from build123d import *

# Parameters (mm, degrees)
F0_W      = 84
F0_H      = 84
F1_DEPTH  = 27
F2_T      = -2.5
F3_DEPTH  = 2
F4_W      = 65
F4_H      = 14
F5_DEPTH  = 25
F6_W      = 10
F6_H      = 10
F7_DEPTH  = 21.8
F4_R      = 2
F8_DEPTH  = 25
F9_DEPTH  = 2
F10_R     = 3.5
F10_R_2   = 1.8
F11_DEPTH = 21
F12_DEPTH = 10
F13_R     = 1
F14_DEPTH = 2
F15_R     = 3


# Not quite as in the source:
# - a feature names something its author has since deleted; it is built from what else it names


with BuildPart() as f1:
    # F0 (on Top) → F1 (new body)
    with BuildSketch(Plane.XY):
        Rectangle(F0_W, F0_H)
    extrude(amount=F1_DEPTH)

    # F2
    f2_openings = [f1.faces().sort_by_distance(p)[0] for p in [
        (0, 0, 27),
    ]]
    offset(amount=F2_T, openings=f2_openings)

    # F3 (cut): a face of the model
    f3_faces = [f1.faces().sort_by_distance(p)[0] for p in [
        (0, 0, 2.5),
    ]]
    extrude(f3_faces, amount=F3_DEPTH, mode=Mode.SUBTRACT)

    # F4 (on face) → F5 (cut)
    with BuildSketch(Plane.XY.offset(2.5)):
        with Locations((0, -27)):
            Rectangle(F4_W, F4_H)
    extrude(amount=-F5_DEPTH, mode=Mode.SUBTRACT)

    # F6 (on face) → F7 (cut)
    with BuildSketch(Plane.YZ.offset(42)):
        with Locations((-27, 5)):
            Rectangle(F6_W, F6_H)
    extrude(amount=-F7_DEPTH, mode=Mode.SUBTRACT)

    # F4 (on face) → F8 (cut)
    with BuildSketch(Plane.XY.offset(2.5)):
        with Locations((0, 26.6423244029)):
            Circle(F4_R)
        with Locations((0, -10.8067262918)):
            Circle(F4_R)
    extrude(amount=-F8_DEPTH, mode=Mode.SUBTRACT)

    # F9 (cut): faces of the model
    f9_faces = [f1.faces().sort_by_distance(p)[0] for p in [
        (0, 40.8120606076, 27),
        (-0.4812956241, 5.0155977429, 2.5),
    ]]
    extrude(f9_faces, amount=-F9_DEPTH, mode=Mode.SUBTRACT)

    # F10 (on Top) → F11 (join)
    with BuildSketch(Plane.XY):
        with Locations((-31.5, 0)):
            Circle(F10_R)
        with Locations((-31.5, 0)):
            Circle(F10_R_2, mode=Mode.SUBTRACT)
        with Locations((31.5, 0)):
            Circle(F10_R)
        with Locations((31.5, 0)):
            Circle(F10_R_2, mode=Mode.SUBTRACT)
    extrude(amount=F11_DEPTH)

    # F10 (on Top) → F12 (join)
    with BuildSketch(Plane.XY):
        with Locations((-31.5, 0)):
            Circle(F10_R_2)
        with Locations((31.5, 0)):
            Circle(F10_R_2)
    extrude(amount=F12_DEPTH)

    # F13
    f13_edges = [f1.edges().sort_by_distance(p)[0] for p in [
        (-42, 42, 12.5),
        (42, 42, 12.5),
        (42, -42, 12.5),
        (-42, -42, 12.5),
    ]]
    fillet(f13_edges, radius=F13_R)

    # F14 (add): a face of the model
    f14_faces = [f1.faces().sort_by_distance(p)[0] for p in [
        (-0.5873435355, 4.470699491, 0),
    ]]
    extrude(f14_faces, amount=F14_DEPTH)

    # F15
    f15_edges = [f1.edges().sort_by_distance(p)[0] for p in [
        (-35, 0, 0.5),
        (28, 0, 0.5),
    ]]
    fillet(f15_edges, radius=F15_R)


solid = f1.part
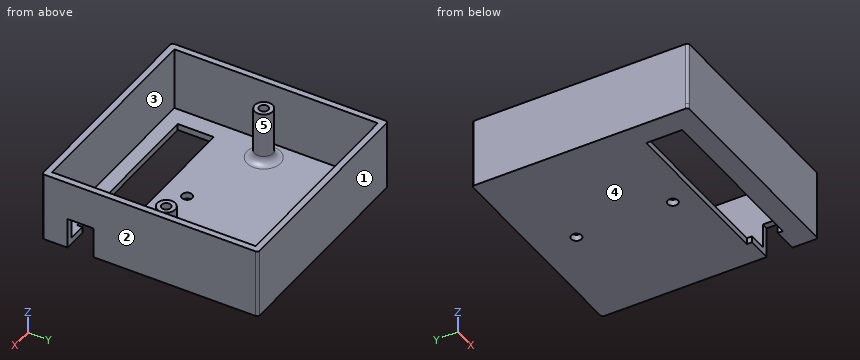
Can you work these out from the model? Positions are in its coordinate system, mm. Face numbers are marked on the shaded views. A direction names the side the tool comes from. Coordinates: 2 decimals unless noted, no trailing zeros. Loops run counter-clockwise (first coordinate to the right, second up) from the corner with the lowest first, then second, coordinate; pieces in that order, holes last. Notation, with made-up numbers: (25.25, 23) - (50.25, 23) arc R21 ccw to (50.25, 29) - close; hole circle Ø4 at (45, 26.5). An arc over 180 degrees is marked (long way). Answer as a JSON object with one key per item and string values. Group by question number.
Item 1: If we section it at D-D (y = -26): List the corners of the cut face in (x, z) for me.
Item 2: For pin 1 (23.5 mm diameter, centred on x = -1.5, y = 19.5, fed in from +Z); pin 2 (2 mm diameter, centred on x = 33, y = 1.5, fed in from +Z); pin 3 (1.1 mm diameter, centred on x = -31.5, y = 0.5, fed in from +Z), each with a flat end and sliding along its axis, tell me the tip position at first contact or that it passes through.
Item 3: If we mould it in two halves opening along Y, with no side actions, what happens to the marked faces 1, 2 and 3? For each: released by +Y, released by -Y, zero draft, split by the parting line, or undercut.
Item 4: If we section it at C-C (x = -31.5): List the corners of the cut face in (y, z) for me.
Item 5: On a 3-axis mill with a long thin cutter (end or side, diameter ignored), from which of +Z, -Z, +X, -X, +Y, -Y can I reach the whole of each face in a straight line? I mean the marked faces 4 and 5. Say none if no direction works.
Item 6: If we section it at A-A (z = 15.5): List the corners of the cut face in (x, y) for me, plus the area to 3 significant figures.
Item 7: If we section it at B-B (x = 0): List the corners of the cut face in (y, z) for me.
Item 8: If I drill on L1, parallel to Y at x = 0, z = -0.95; L2, parallel to Y at x = -31.5, z = 14.25; L3, parallel to Y at x = 24, z = 17.25, over which ranges is the centre line in solid material (lowest first)? Write a range as from..to.
Returned:
{
 "1": {"outline": "(-42, -2) - (-32.5, -2) - (-32.5, 0.5) - (-39.5, 0.5) - (-39.5, 25) - (-42, 25) - close; (39.5, 10) - (42, 10) - (42, 25) - (39.5, 25) - close"},
 "2": {"pin 1": "stops at z = 0.5", "pin 2": "stops at z = 21", "pin 3": "stops at z = 10"},
 "3": {"face 1": "released by +Y", "face 2": "zero draft", "face 3": "undercut"},
 "4": {"outline": "(-42, -2) - (-34, -2) - (-34, 0.5) - (-39.5, 0.5) - (-39.5, 25) - (-42, 25) - close; (-20, -2) - (42, -2) - (42, 25) - (39.5, 25) - (39.5, 0.5) - (6.5, 0.5) arc R3 cw to (3.5, 3.5) - (3.5, 21) - (1.8, 21) - (1.8, 10) - (-1.8, 10) - (-1.8, 21) - (-3.5, 21) - (-3.5, 3.5) arc R3 cw to (-6.5, 0.5) - (-20, 0.5) - close"},
 "5": {"face 4": "-Z, +X, -X, +Y, -Y", "face 5": "+Z"},
 "6": {"outline": "(-42, -41) arc R1 ccw to (-41, -42) - (41, -42) arc R1 ccw to (42, -41) - (42, 41) arc R1 ccw to (41, 42) - (-41, 42) arc R1 ccw to (-42, 41) - close; circle Ø7 at (-31.5, 0); circle Ø7 at (31.5, 0); hole (-39.5, -39.5) - (39.5, -39.5) - (39.5, 39.5) - (-39.5, 39.5) - close; hole circle Ø3.6 at (-31.5, 0); hole circle Ø3.6 at (31.5, 0)", "area": "871 mm²"},
 "7": {"outline": "(-42, -2) - (-34, -2) - (-34, 0.5) - (-39.5, 0.5) - (-39.5, 25) - (-42, 25) - close; (-20, -2) - (-12.81, -2) - (-12.81, 0.5) - (-20, 0.5) - close; (-8.81, -2) - (24.64, -2) - (24.64, 0.5) - (-8.81, 0.5) - close; (28.64, -2) - (42, -2) - (42, 25) - (39.5, 25) - (39.5, 0.5) - (28.64, 0.5) - close"},
 "8": {"L1": "y = -42..-34, -20..-12.81, -8.81..24.64, 28.64..42", "L2": "y = -42..-39.5, -3.5..-1.8, 1.8..3.5, 39.5..42", "L3": "y = -42..-39.5, 39.5..42"}
}
